```python
from build123d import *

# Parameters (mm, degrees)
F2_R     = 1.984375
F3_DEPTH = 7.725815
F4_ANGLE = 180


with BuildPart() as f1:
    # F0 (on Front) → F1 (revolve)
    with BuildSketch(Plane.XZ):
        Polygon((13.5, -4.549815), (14.29375, -3.175), (14.29375, 0), (14.29375, 3.175), (0, 3.175), (0, 0), (12.70625, 0), (12.70625, -3.175), align=None)
    revolve(axis=Axis((0, 0, -9.971488), (0, 0, -1)))

    # F2 (on face) → F3 (cut, through all)
    with BuildSketch(Plane.XY.offset(3.175)):
        Circle(F2_R)
    extrude(amount=-F3_DEPTH, mode=Mode.SUBTRACT)


with BuildPart() as f1_1:
    # F4: moved
    add(f1.part.rotate(Axis((-6.353125, 0, 0), (1, 0, 0)), F4_ANGLE))


solid = f1_1.part
```
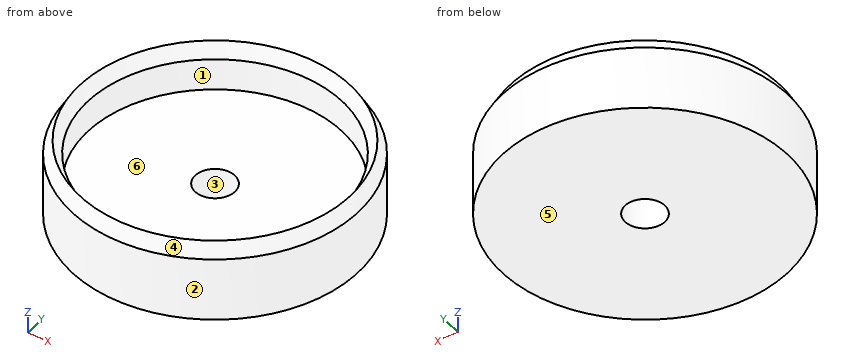
Check sheet for the modelled part. Datum: model origin and axes. Units: mm. Face numbers are marked on the shaded views. A direction names the side the tool comes from. Round coordinates to 2 decimals unless told otherwise and drop trailing zeros. Order: outer loops, then holes, each group sorted by start corner. A loop starts at its lowest first (then second) coordinate and runs counter-clockwise, first axis right, second up. Notation, with made-up numbers: (84.5, 13) - (132.5, 13) arc R29 ccw to (132.5, 48) - close; hole circle Ø6 at (-14.5, 57.25). An arc over 180 degrees is marked (long way). Answer as CSV lines item,"result". Start each with the question number.
1) Section check C-C (z = 2.25). Record the cut outline in (x, y), then the cut area to 3 significant figures.
2) Section check A-A (y = 0). Record the cut outline in (x, z) (3 decimals), then the cut area to 3 significant figures.
3) Depth check by flat-ended pin: pin 1 (6 mm diameter, centred on x = 4, y = -10.5, fed in from +Z); pin 2 (3.5 mm diameter, centred on x = 0, y = 0, fed in from -Z); pin 3 (2 mm diameter, centred on y = 5, z = -1.5, fed in from -X); pin 4 (2 mm diameter, centred on x = -8, y = 7.5, fed in from +Z). Enter the tip coordinate at first touch or a pass-through.
4) Scan lines: probe 1 along Y at (x, z) = (0, -0.7); probe 2 along Z at (x, y) = (-12, 0) (3 decimals); probe 3 along Y at (x, z) = (3.75, 3.5). Record each from-to range of solid material in increasing order.
5) Draft check along X on the marked faces 3, 4, 5 and 6. Enter one of: +X half, -X half, draft (parallel to the pull), parting line (faces both ways), or undercut.
6) Tool access check on the marked faces 1 and 2. Record the directions out of +Z, -Z, +X, -X, +Y, -Y that give a thin tool (end or side, any length) a straight path to the whole face; none if there is none.
Determined:
1,outline,"circle Ø28.59 at (0, 0); hole circle Ø25.41 at (0, 0)"
1,area,"135 mm^2"
2,outline,"(-14.294, -3.175) - (-1.984, -3.175) - (-1.984, 0) - (-12.706, 0) - (-12.706, 3.175) - (-13.5, 4.55) - (-14.294, 3.175) - close; (1.984, -3.175) - (14.294, -3.175) - (14.294, 3.175) - (13.5, 4.55) - (12.706, 3.175) - (12.706, 0) - (1.984, 0) - close"
2,area,"90.4 mm^2"
3,pin 1,"z = 4.55"
3,pin 2,"through"
3,pin 3,"x = -13.72"
3,pin 4,"z = 0"
4,probe 1,"-14.29 to -1.98, 1.98 to 14.29"
4,probe 2,"-3.175 to 0"
4,probe 3,"-13.6 to -12.34, 12.34 to 13.6"
5,face 3,"undercut"
5,face 4,"parting line"
5,face 5,"draft"
5,face 6,"undercut"
6,face 1,"+Z"
6,face 2,"+Z, -Z"
